For this review, take the finished solid that the model builds, in its own axes (mm). Face numbers are marked on the shaded views. A direction names the side the tool comes from. Coordinates: 2 decimals unless noted, no trailing zeros. Order: outer loops, then holes, each group sorted by start corner. A loop starts at its lowest first (then second) coordinate and runs counter-clockwise, first axis right, second up. Notation, with made-up numbers: (26.25, -35.5) -> (41.25, -35.5) arc R10 cw to (41.25, -18.5) -> close; hole circle Ø6 at (68, 72). An arc over 180 degrees is marked (long way). Return JSON: item names as keys, results as strings. Group by question number.
Item 1: Take a section at B-B (y = -5). Write out the cut boundary in (x, z), then the cut area to 3 significant figures.
Item 2: Insertion check: pin 1 (4 mm diameter, centred on y = -4, z = 9, fed in from -X); pin 2 (2.5 mm diameter, centred on x = 6, y = -0.5, fed in from +Z); pin 3 (6.5 mm diameter, centred on x = 5.13, y = 0, fed in from +Z). Each pin has a flat end and moves straight along its axis. Give the tip position at first contact, or say it passes through.
Item 3: Take a section at D-D (x = 1.5). Write out the cut boundary in (y, z), then the cut area to 3 significant figures.
Item 4: Draft analysis for pull direction Y (two halves, no side actions). For the marked faces 1, 2 and 3, state which applies: +Y half, -Y half, draft (parallel to the pull), parting line (faces both ways), or undercut.
Item 5: Machinability: for the marked faces 4, 5 and 6, which of the approach directions +Z, -Z, +X, -X, +Y, -Y give a long, thin tool a straight path to every point of the face, cutting with its end or side? Answer none if there is none.
Item 6: For line 1 along Z through (x, y) = (2.5, -4.75); line 2 along Z through (x, y) = (-2.5, 3.5); line 3 along X through (y, z) = (5, 9.75), list the stretches that pass through material, from the lowest coordinate up.
Item 7: Take a section at A-A (y = 0). Write out the cut boundary in (x, z).
Item 8: Take a section at C-C (z = 4.5). Write out the cut boundary in (x, y), then the cut area to 3 significant figures.
```python
from build123d import *

# Parameters (mm, degrees)
F1_DEPTH  = 2.8
F2_R      = 3
F3_SIZE   = 1
F1_FACE_W = 25
F1_FACE_H = 2.8
F4_DEPTH  = 1.5
F5_W      = 2.63875
F5_H      = 25
F6_DEPTH  = 12.7
F7_W      = 25
F7_H      = 1.989666
F8_DEPTH  = 3


with BuildPart() as f1:
    # F0 (on Top) → F1 (new body)
    with BuildSketch(Plane.XY):
        with BuildLine():
            Line((9.196268, 0), (7.12831, 0))
            ThreePointArc((7.12831, 0), (5.12831, -2), (3.12831, 0))
            Line((3.12831, 0), (0, 0))
            Line((0, 0), (0, -12.5))
            Line((0, -12.5), (3, -12.5))
            Line((3, -12.5), (9.196268, 0))
        make_face()
        with BuildLine():
            ThreePointArc((3.12831, 0), (5.12831, 2), (7.12831, 0))
            Line((7.12831, 0), (9.196268, 0))
            Line((9.196268, 0), (3, 12.5))
            Line((3, 12.5), (0, 12.5))
            Line((0, 12.5), (0, 0))
            Line((0, 0), (3.12831, 0))
        make_face()
    extrude(amount=F1_DEPTH)

    # F2
    f2_edges = [f1.edges().sort_by_distance(p)[0] for p in [
        (9.196268, 0, 1.4),
        (3, -12.5, 1.4),
        (3, 12.5, 1.4),
    ]]
    fillet(f2_edges, radius=F2_R)

    # F3
    f3_edges = [f1.edges().sort_by_distance(p)[0] for p in [
        (3.12831, 0, 2.8),
    ]]
    chamfer(f3_edges, length=F3_SIZE)

    # F1_face (on face) → F4 (join)
    with BuildSketch(Plane(origin=(0, 0, 1.4), x_dir=(0, -1, 0), z_dir=(-1, 0, 0))):
        Rectangle(F1_FACE_W, F1_FACE_H)
    extrude(amount=F4_DEPTH)

    # F5 (on face) → F6 (join)
    with BuildSketch(Plane.XY.offset(2.8)):
        with Locations((-0.180625, 0)):
            Rectangle(F5_W, F5_H)
    extrude(amount=F6_DEPTH)

    # F7 (on face) → F8 (join)
    with BuildSketch(Plane(origin=(-1.5, 0, 0), x_dir=(0, -1, 0), z_dir=(-1, 0, 0))):
        with Locations((0, 14.505167)):
            Rectangle(F7_W, F7_H)
    extrude(amount=F8_DEPTH)


solid = f1.part
```
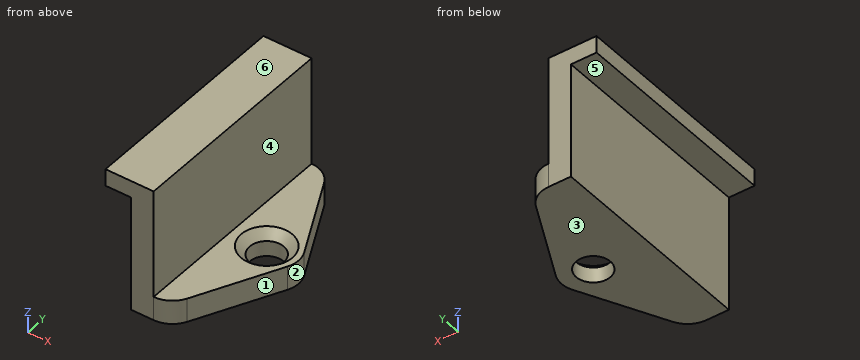
Findings below:
{
 "1": {"outline": "(-4.5, 13.51) -> (-1.5, 13.51) -> (-1.5, 0) -> (6.72, 0) -> (6.72, 2.8) -> (1.14, 2.8) -> (1.14, 15.5) -> (-4.5, 15.5) -> close", "area": "62.5 mm2"},
 "2": {"pin 1": "stops at x = -1.5", "pin 2": "stops at z = 2.05", "pin 3": "stops at z = 2.8"},
 "3": {"outline": "(-12.48, 0) -> (12.48, 0) -> (12.48, 2.8) -> (-12.48, 2.8) -> close", "area": "69.9 mm2"},
 "4": {"face 1": "-Y half", "face 2": "parting line", "face 3": "draft"},
 "5": {"face 4": "+Z, +X, +Y, -Y", "face 5": "-Z, -X, +Y, -Y", "face 6": "+Z, +X, -X, +Y, -Y"},
 "6": {"line 1": "z = 0 to 2.8", "line 2": "z = 13.51 to 15.5", "line 3": "x = -1.5 to 1.14"},
 "7": {"outline": "(-4.5, 13.51) -> (-1.5, 13.51) -> (-1.5, 0) -> (3.13, 0) -> (3.13, 1.8) -> (2.13, 2.8) -> (1.14, 2.8) -> (1.14, 15.5) -> (-4.5, 15.5) -> close; (7.13, 0) -> (8.85, 0) -> (8.85, 2.8) -> (8.13, 2.8) -> (7.13, 1.8) -> close"},
 "8": {"outline": "(-1.5, -12.5) -> (1.14, -12.5) -> (1.14, 12.5) -> (-1.5, 12.5) -> close", "area": "66.0 mm2"}
}
